Job drawing, mm, ordinate dimensions from the low corner. One solid piece. A direction names the side the tool comes from. Give positions to 0.01 mm unless a question says otherwise; leave off trailing zeros. Order: outer loops, then holes, each group sorted by start corner. A loop starts at its lowest first (then second) coordinate and runs counter-clockwise, first axis right, second up. Notation, with made-up numbers: (16, -3.5) -> (60, -3.5) arc R17 cw to (60, 15.5) -> close; hole circle Ø8 at (27, 67). An arc over 180 degrees is marked (long way). Use CSV: the item, a comma, the result in double quotes. Start each with the question number.
1. Drop flat-ended pins along their axis: pin 1 (8.5 mm diameter, centred on y = 18, z = 67.5, fed in from +X); pin 2 (3 mm diameter, centred on x = 32.5, y = 19, fed in from +Z); pin 3 (10 mm diameter, centred on x = 23, z = 118.5, fed in from +Y); pin 4 (8 mm diameter, centred on x = 35, y = 17.5, fed in from +Z). Give the stop position or say it passes through.
2. Cut at D-D on z = 84.5. List the corners of the cut face in (x, y).
3. 3-axis set-ups, long thin cutter, end or side, ignore diameter. For the marked faces 1, 2 and 3: which of +Z, -Z, +X, -X, +Y, -Y reach the whole face in a straight line?
4. Cut at C-C on y = 13.9. List the corners of the cut face in (x, z), then the cut area to 3 significant figures.
5. Cut at B-B on x = 30. List the corners of the cut face in (y, z).
6. Cut at A-A on x = 20. List the corners of the cut face in (y, z).
7. Wall check: line 1 (X direction, y = 2, z = 67.5); line 2 (Z direction, x = 21.5, y = 12.25); line 3 (Z direction, x = 56.5, y = 14.5). Give the ranges that are in metal, low to high. Write a range as from..to.
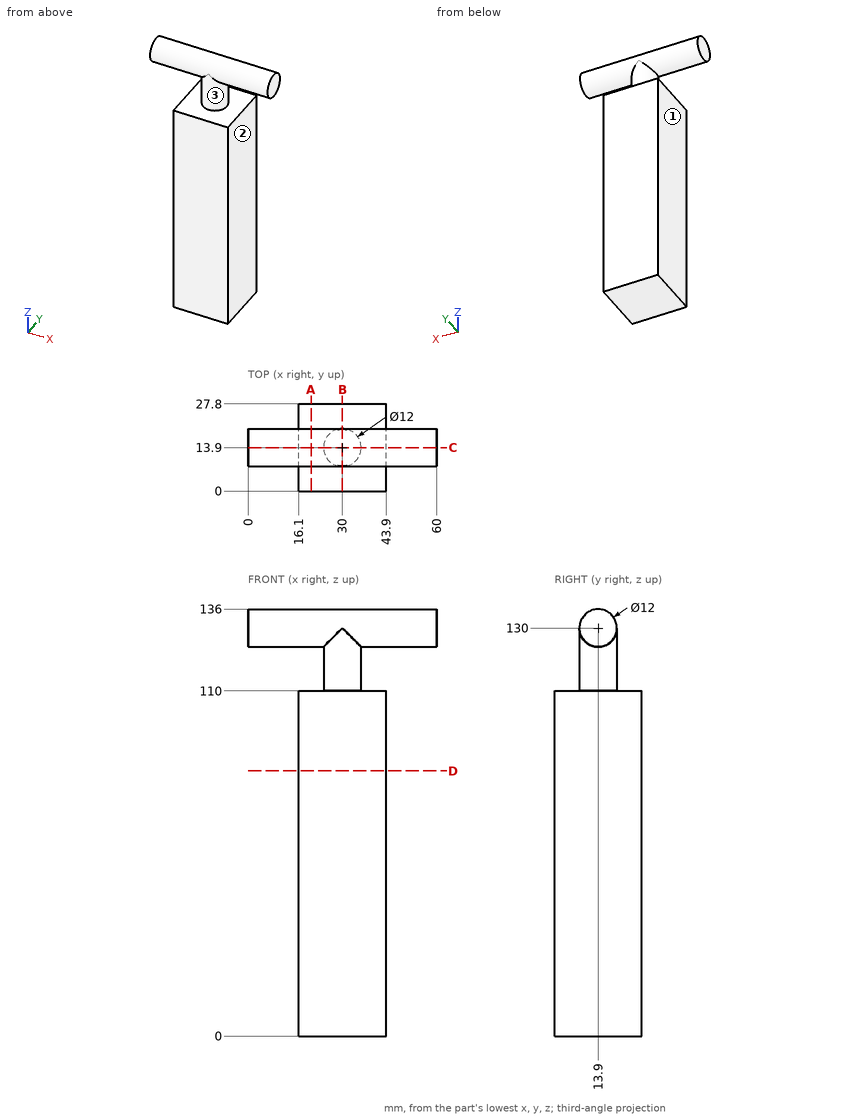
Verdict:
1,pin 1,"x = 43.9"
1,pin 2,"z = 134.8"
1,pin 3,"y = 19.56"
1,pin 4,"z = 136"
2,outline,"(16.1, 0) -> (43.9, 0) -> (43.9, 27.8) -> (16.1, 27.8) -> close"
3,face 1,"-Z, -X, +Y, -Y"
3,face 2,"-Z, +X, +Y, -Y"
3,face 3,"none"
4,outline,"(0, 124) -> (24, 124) -> (24, 110) -> (16.1, 110) -> (16.1, 0) -> (43.9, 0) -> (43.9, 110) -> (36, 110) -> (36, 124) -> (60, 124) -> (60, 136) -> (0, 136) -> close"
4,area,"3,950 mm^2"
5,outline,"(0, 0) -> (27.8, 0) -> (27.8, 110) -> (19.9, 110) -> (19.9, 130) arc R6 ccw to (7.9, 130) -> (7.9, 110) -> (0, 110) -> close"
6,outline,"(0, 0) -> (27.8, 0) -> (27.8, 110) -> (0, 110) -> close; circle Ø12 at (13.9, 130)"
7,line 1,"16.1..43.9"
7,line 2,"0..110, 124.23..135.77"
7,line 3,"124.03..135.97"
